The figure shows three views and two pictorial views of one solid part (mm, origin at its lowest corner). Answer the questions. Coordinates: 2 decimals unless noted, no trailing zeros. Loops run counter-clockwise (first coordinate to the right, second up) from the corner with the lowest first, then second, coordinate; pieces in that order, holes last. Notation, with made-up numbers: (-14, 62) -> (45, 62) arc R24 cw to (45, 84) -> close; hole circle Ø7 at (15.5, -9). An arc over 180 degrees is marked (long way). Answer as a JSON object with one key per item and string values. Group by question number.
1) Section B-B, the plane x = 140.5 is taken. Give the vertices of the cut face in (y, z).
2) Consider probe 1 along Z at (x, y) = (216, 3.65); probe 2 along X at (y, z) = (2.4, 24.5); probe 3 along X at (y, z) = (1.7, 167). Determine where each line is inside the solid, lowest interval first. Write a range as [from, to].
3) Flat-ended cylindrical pins translate along their axes: P1, Ø1.5, axis at y = 3, z = 1.5, coming from the +X side; P2, Ø2, axis at x = 24, z = 165.5, coming from the +Y side; P3, Ø1.5, axis at x = 2, y = 1.5, coming from the +Z side; P4, Ø2.5, axis at y = 3, z = 145.5, coming from the +X side. Find the tip coordinate at first contact, or state that the pin passes through.
4) Section A-A, the plane y = 3.05 is taken. Count the separate pieces of the cut face and the enclosed holes in it, plus the area to 3 significant figures.
5) Section C-C, the plane z = 157 is taken. Give the vertices of the cut face in (x, y), plus the area to 3 significant figures.
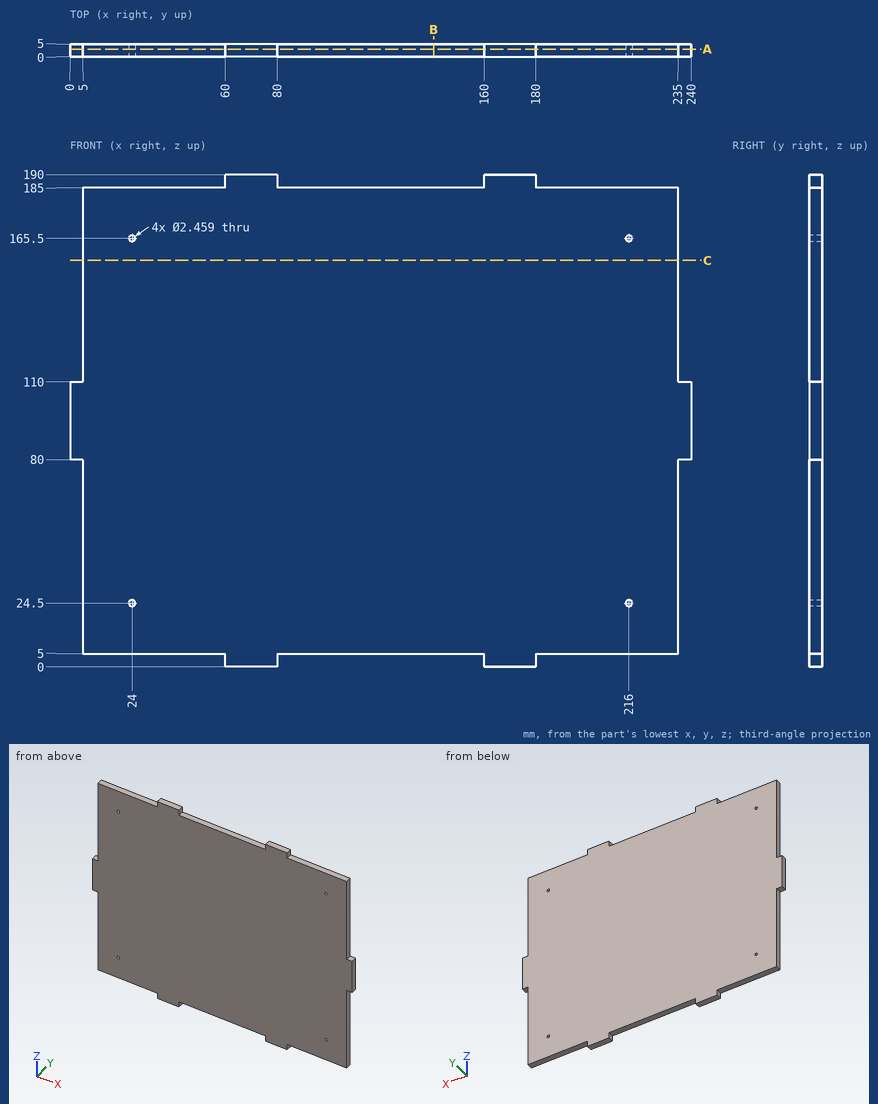
Determined:
{
 "1": {"outline": "(0, 5) -> (5, 5) -> (5, 185) -> (0, 185) -> close"},
 "2": {"probe 1": "[5, 23.27], [25.73, 164.27], [166.73, 185]", "probe 2": "[5, 22.77], [25.23, 214.77], [217.23, 235]", "probe 3": "[5, 235]"},
 "3": {"P1": "x = 180", "P2": "through", "P3": "z = 110", "P4": "x = 235"},
 "4": {"separate pieces": "1", "enclosed holes": "4", "area": "42,100 mm²"},
 "5": {"outline": "(5, 0) -> (235, 0) -> (235, 5) -> (5, 5) -> close", "area": "1,150 mm²"}
}
